Work out the finished part from the listing and answer in its coordinate system (mm). Face numbers are marked on the shaded views. Coordinates: 2 decimals unless noted, no trailing zeros. Order: outer loops, then holes, each group sorted by start corner. A loop starts at its lowest first (then second) coordinate and runs counter-clockwise, first axis right, second up.
1. The part is cut by section B-B, the plane z = 5.75. Give the vertices of the cut face in (x, y) (1 decimal), then the cut area to 3 significant figures.
2. The part is cut by section C-C, the plane y = -1.1. Give the vertices of the cut face in (x, z).
3. Find the intervals of material crossed by probe 1 along X at (y, z) = (0, 3.2) (1 decimal); probe 2 along Y at (x, z) = (0.65, 4.5), in increasing order.
4. Flat-ended cylindrical pins translate along their axes: pin 1 Ø0.9 at (x, z) = (1, 0.5) entering from +Y; pin 2 Ø2 at (x, y) = (0.5, 0) entering from +Z. Find the tip coordinate at first contact, or state that the pin passes through.
5. Determine the mould class of the marked faces 1, 2 and 3 for opening direction Y: +Y half, -Y half, draft (parallel to the pull), parting line (faces both ways), or undercut.
6. The part is cut by section A-A, the plane x = -0.85. Give the vertices of the cut face in (y, z), then the cut area to 3 significant figures.
7. The part is cut by section D-D, the plane x = -1.5. Give the vertices of the cut face in (y, z), then the cut area to 3 significant figures.
```python
from build123d import *

# Parameters (mm, degrees)
F0_R     = 2.2225
F1_DEPTH = 6.35
F2_R     = 1.905
F3_DEPTH = 4.572
F5_DEPTH = 2.2235


with BuildPart() as f1:
    # F0 (on Top) → F1 (new body)
    with BuildSketch(Plane.XY):
        Circle(F0_R)
    extrude(amount=F1_DEPTH)

    # F2 (on face) → F3 (cut)
    with BuildSketch(Plane.XY.offset(6.35)):
        Circle(F2_R)
    extrude(amount=-F3_DEPTH, mode=Mode.SUBTRACT)

    # F4 (on Front) → F5 (cut, through all)
    with BuildSketch(Plane.XZ):
        Polygon((0, 2.811728), (-2.906317, 0), (3.048, 0), align=None)
    extrude(amount=-F5_DEPTH, mode=Mode.SUBTRACT)


solid = f1.part
```
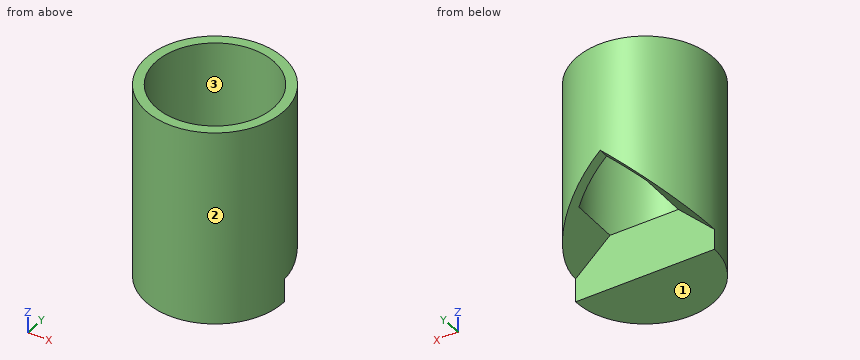
Geometry says:
1. outline: circle Ø4.4 at (0, 0); hole circle Ø3.8 at (0, 0)
1. area: 4.12 mm2
2. outline: (-1.93, 0) - (1.93, 0) - (1.93, 6.35) - (1.56, 6.35) - (1.56, 1.78) - (-1.56, 1.78) - (-1.56, 6.35) - (-1.93, 6.35) - close
3. probe 1: x = -2.2 to -1.9, 1.9 to 2.2
3. probe 2: y = -2.13 to -1.79, 1.79 to 2.13
4. pin 1: stops at y = 0
4. pin 2: stops at z = 1.78
5. face 1: draft
5. face 2: parting line
5. face 3: undercut
6. outline: (-2.05, 0) - (0, 0) - (0, 1.78) - (-1.7, 1.78) - (-1.7, 6.35) - (-2.05, 6.35) - close; (1.7, 1.99) - (2.05, 1.99) - (2.05, 6.35) - (1.7, 6.35) - close
6. area: 6.77 mm2
7. outline: (-1.64, 0) - (0, 0) - (0, 1.36) - (1.64, 1.36) - (1.64, 6.35) - (1.17, 6.35) - (1.17, 1.78) - (-1.17, 1.78) - (-1.17, 6.35) - (-1.64, 6.35) - close
7. area: 7.86 mm2
